```python
from build123d import *

# Parameters (mm, degrees)
F1_DEPTH = 2.5
F2_R     = 0.85
F3_DEPTH = 12.5


with BuildPart() as f1:
    # F0 (on Top) → F1 (new body)
    with BuildSketch(Plane.XY):
        with BuildLine():
            Line((13.081475452, -13.081475452), (1.0606601718, -1.0606601718))
            ThreePointArc((1.0606601718, -1.0606601718), (0, -0.6213203436), (-1.0606601718, -1.0606601718))
            Line((-1.0606601718, -1.0606601718), (-13.081475452, -13.081475452))
            ThreePointArc((-13.081475452, -13.081475452), (-13.5208152802, -14.1421356237), (-13.081475452, -15.2027957955))
            Line((-13.081475452, -15.2027957955), (-1.0606601718, -27.2236110757))
            ThreePointArc((-1.0606601718, -27.2236110757), (0, -27.6629509039), (1.0606601718, -27.2236110757))
            Line((1.0606601718, -27.2236110757), (13.081475452, -15.2027957955))
            ThreePointArc((13.081475452, -15.2027957955), (13.5208152802, -14.1421356237), (13.081475452, -13.081475452))
        make_face()
        with BuildLine():
            Line((-5.9082568333, -12.0771760074), (-5.9082568333, -7.1194937158))
            Line((-5.9082568333, -7.1194937158), (-4.5074321806, -7.1194937158))
            add(Edge.make_bspline(
                [(-4.5074321806, -7.1194937158), (-3.5211040556, -7.1194937158), (-3.0800233264, -7.4146326047)],
                knots=[0, 0, 0, 1, 1, 1], degree=2))
            add(Edge.make_bspline(
                [(-3.0800233264, -7.4146326047), (-2.6389425972, -7.7097714936), (-2.6389425972, -8.3467072574)],
                knots=[0, 0, 0, 1, 1, 1], degree=2))
            add(Edge.make_bspline(
                [(-2.6389425972, -8.3467072574), (-2.6389425972, -8.7883305213), (-2.8847108264, -9.0747888547)],
                knots=[0, 0, 0, 1, 1, 1], degree=2))
            add(Edge.make_bspline(
                [(-2.8847108264, -9.0747888547), (-3.1304790556, -9.361247188), (-3.6024842639, -9.4458826047)],
                knots=[0, 0, 0, 1, 1, 1], degree=2))
            Line((-3.6024842639, -9.4458826047), (-3.6024842639, -9.4795197574))
            add(Edge.make_bspline(
                [(-3.6024842639, -9.4795197574), (-2.4729269722, -9.6726621186), (-2.4729269722, -10.6665857297)],
                knots=[0, 0, 0, 1, 1, 1], degree=2))
            add(Edge.make_bspline(
                [(-2.4729269722, -10.6665857297), (-2.4729269722, -11.3306482297), (-2.9221457222, -11.7039121186)],
                knots=[0, 0, 0, 1, 1, 1], degree=2))
            add(Edge.make_bspline(
                [(-2.9221457222, -11.7039121186), (-3.3713644722, -12.0771760074), (-4.1786561389, -12.0771760074)],
                knots=[0, 0, 0, 1, 1, 1], degree=2))
            Line((-4.1786561389, -12.0771760074), (-5.9082568333, -12.0771760074))
        make_face(mode=Mode.SUBTRACT)
        with BuildLine():
            Line((-8.1334756687, -14.8039748892), (-8.1334756687, -13.4802963582))
            Line((-8.1334756687, -13.4802963582), (-0.6236797201, -13.4802963582))
            Line((-0.6236797201, -13.4802963582), (-0.6236797201, -6.9198086858))
            ThreePointArc((-0.6236797201, -6.9198086858), (-0.9032194318, -6.4583786209), (-0.9135835525, -5.9189782686))
            ThreePointArc((-0.9135835525, -5.9189782686), (0.0168397474, -5.0141534426), (0.9868078824, -5.876451129))
            ThreePointArc((0.9868078824, -5.876451129), (0.9900106564, -6.4384308628), (0.6999988109, -6.9198086858))
            Line((0.6999988109, -6.9198086858), (0.6999988109, -13.4802963582))
            Line((0.6999988109, -13.4802963582), (8.1334756687, -13.4802963582))
            ThreePointArc((8.1334756687, -13.4802963582), (8.5949057336, -13.2007566465), (9.134306086, -13.1903925258))
            ThreePointArc((9.134306086, -13.1903925258), (10.0391309119, -14.1208158258), (9.1768332255, -15.0907839607))
            ThreePointArc((9.1768332255, -15.0907839607), (8.6148534917, -15.0939867347), (8.1334756687, -14.8039748892))
            Line((8.1334756687, -14.8039748892), (0.6999988109, -14.8039748892))
            Line((0.6999988109, -14.8039748892), (0.6999988109, -23.1867600232))
            Line((0.6999988109, -23.1867600232), (-0.6236797201, -23.1867600232))
            Line((-0.6236797201, -23.1867600232), (-0.6236797201, -14.8039748892))
            Line((-0.6236797201, -14.8039748892), (-8.1334756687, -14.8039748892))
        make_face(mode=Mode.SUBTRACT)
        with BuildLine():
            add(Edge.make_bspline(
                [(5.6933566328, -7.7602282705), (6.3340901397, -8.4009617774), (6.3340901397, -9.5511353885)],
                knots=[0, 0, 0, 1, 1, 1], degree=2))
            add(Edge.make_bspline(
                [(6.3340901397, -9.5511353885), (6.3340901397, -10.7783489302), (5.6678575008, -11.4277629927)],
                knots=[0, 0, 0, 1, 1, 1], degree=2))
            add(Edge.make_bspline(
                [(5.6678575008, -11.4277629927), (5.0016248619, -12.0771770552), (3.7505397925, -12.0771770552)],
                knots=[0, 0, 0, 1, 1, 1], degree=2))
            Line((3.7505397925, -12.0771770552), (2.3768418758, -12.0771770552))
            Line((2.3768418758, -12.0771770552), (2.3768418758, -7.1194947635))
            Line((2.3768418758, -7.1194947635), (3.8959390981, -7.1194947635))
            add(Edge.make_bspline(
                [(3.8959390981, -7.1194947635), (5.0526231258, -7.1194947635), (5.6933566328, -7.7602282705)],
                knots=[0, 0, 0, 1, 1, 1], degree=2))
        make_face(mode=Mode.SUBTRACT)
    extrude(amount=F1_DEPTH)

    # F2 (on Right) → F3 (cut, symmetric)
    with BuildSketch(Plane.YZ):
        with Locations((-2.4908210296, 1.292226194)):
            Circle(F2_R)
    extrude(amount=F3_DEPTH, both=True, mode=Mode.SUBTRACT)


solid = f1.part
```
Build history of the part. All positions in model axes, mm. A direction names the side the tool comes from. Round coordinates to 2 decimals unless told otherwise and drop trailing zeros. Order: outer loops, then holes, each group sorted by start corner. A loop starts at its lowest first (then second) coordinate and runs counter-clockwise, first axis right, second up. Notation, with made-up numbers: (-23, -24) -> (34, -24) arc R6 cw to (34, -17) -> close; hole circle Ø1 at (68, -22.5). An arc over 180 degrees is marked (long way). Answer in a Markdown table with one row per item.
1) Band-saw the part on C-C on y = -11.25. Give the number of separate pieces and of enclosed holes in the cut face, and give its area (3 significant figures).
Values:
| item | result |
|---|---|
| separate pieces | 4 |
| enclosed holes | 0 |
| area | 36.0 mm2 |
2) Band-saw the part on A-A on x = -7.75. Give the cut face in (y, z), and give its area (3 significant figures).
Values:
| item | result |
|---|---|
| outline | (-20.53, 0) -> (-14.8, 0) -> (-14.8, 2.5) -> (-20.53, 2.5) -> close; (-13.48, 0) -> (-7.75, 0) -> (-7.75, 2.5) -> (-13.48, 2.5) -> close |
| area | 28.7 mm2 |
3) Band-saw the part on B-B on y = -18.25. Give the cut face in (x, z).
Values:
| item | result |
|---|---|
| outline | (-10.03, 0) -> (-0.62, 0) -> (-0.62, 2.5) -> (-10.03, 2.5) -> close; (0.7, 0) -> (10.03, 0) -> (10.03, 2.5) -> (0.7, 2.5) -> close |
4) Mould opens along X. For faces 1 (the flat face through (1, -16, 2.5)), 2 (the cylindrical face through (-0.016, -27.663, 1.232)), 3 (the flat face through (-5.908, -10, 1)), 4 (the cylindrical face through (8.623, -15.096, 1.232)) say: released by +X, released by -X, zero draft, split by the parting line, or undercut.
Values:
| item | result |
|---|---|
| face 1 | zero draft |
| face 2 | split by the parting line |
| face 3 | undercut |
| face 4 | undercut |
5) Pin check, flat tips, straight feed: P1, Ø1.5, axis at x = -2, z = 0.5, coming from the -Y side; P2, Ø1.1, axis at y = -14, z = 1.5, coming from the +X side; P3, Ø1.5, axis at x = -5.5, z = 1, coming from the -Y side; P4, Ø0.8, axis at y = -17.5, z = 1, coming from the +X side. Stop position of each tip, or through.
Values:
| item | result |
|---|---|
| P1 | y = -27.03 |
| P2 | x = 13.52 |
| P3 | y = -23.53 |
| P4 | x = 11.18 |
6) Which spindle directions (+Z, -Z, +X, -X, +Y, -Y) get a long thin tool onto all of the face, cutting with end or side? Do faces 5 (the flat face through (1, -16, 0)), 6 (the flat face through (0.7, -10, 1)). Say none if no direction does.
Values:
| item | result |
|---|---|
| face 5 | -Z, +X, -X, +Y, -Y |
| face 6 | +Z, -Z |
7) Band-saw the part on D-D on x = 11.75. Give the cut face in (y, z), and give its area (3 significant figures).
Values:
| item | result |
|---|---|
| outline | (-16.53, 0) -> (-11.75, 0) -> (-11.75, 2.5) -> (-16.53, 2.5) -> close |
| area | 12.0 mm2 |
8) Wall check: L1, parallel to Y at x = 4.75, z = 2.25; L2, parallel to X at y = -11.25, z = 0.5; L3, parallel to Y at x = -5, z = 0.45. Give the ranges that are in metal, low to high.
Values:
| item | result |
|---|---|
| L1 | -23.53 to -14.8, -13.48 to -11.95, -7.23 to -4.75 |
| L2 | -11.25 to -5.91, -2.58 to -0.62, 0.7 to 2.38, 5.83 to 11.25 |
| L3 | -23.28 to -14.8, -13.48 to -12.08, -7.12 to -5 |
